Geometry: final body of the model. Coordinates: model frame, mm. Face numbers are marked on the shaded views. A direction names the side the tool comes from. Give positions to 0.01 mm unless a question says otherwise; leave off trailing zeros. Loops run counter-clockwise (first coordinate to the right, second up) from the corner with the lowest first, then second, coordinate; pieces in that order, holes last. Notation, with made-up numbers: (-20, 29.25) -> (18, 29.25) arc R21 ccw to (18, 60.25) -> close; hole circle Ø4 at (-4.5, -25.75). An arc over 180 degrees is marked (long way). One line per question, with ' | ' between items. Start each with the question number.
Item 1: Material intervals for line 1 along X through (y, z) = (8.75, -11.5); line 2 along X through (y, z) = (5.5, 0); line 3 along X through (y, z) = (8, -10), sorted ascending. Write a range as [from, to].
Item 2: Section B-B on x = 20.75. Return loops of the section in (y, z).
Item 3: Section D-D on z = 9.75. Return loops of the section in (x, y), then the cut area to 3 significant figures.
Item 4: Mould query, pull axis Z, two halves, no side actions, for the marked faces 1, 2, 3 and 4. Classes: released by +Z, released by -Z, zero draft, split by the parting line, or undercut.
Item 5: Section A-A on y = 6.5. Return loops of the section in (x, z).
Item 6: Section C-C on z = -1.75. Return loops of the section in (x, y), then the cut area to 3 significant figures.
Item 7: Set-up query: the marked faces 5, 6 and 7. Return all of +Z, -Z, +X, -X, +Y, -Y with unobstructed straight access to the full face (end or side cutting, diameter ignored); none if empty.
Item 8: Pin query (flat end, axial travel): P1, Ø3, axis at y = 11, z = -10.5, coming from the -X side; P2, Ø2.5, axis at y = 9.5, z = -6.5, coming from the -X side; P3, Ø3, axis at y = 11, z = 3.5, coming from the -X side; P4, Ø6.5, axis at x = 18.5, y = 8.5, coming from the +Z side. Return the tip coordinate at first contact, or that it passes through.
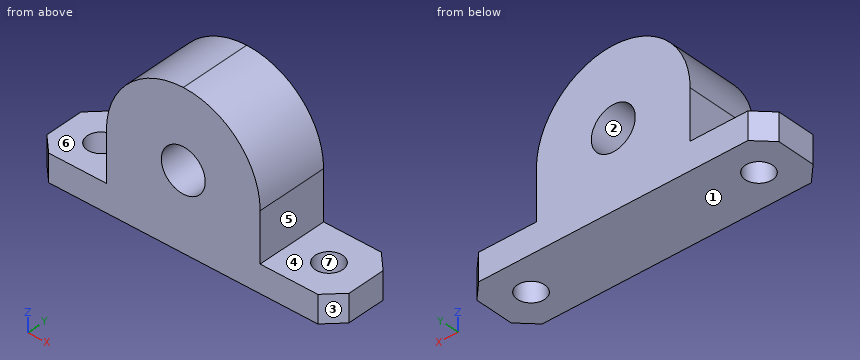
from build123d import *

# Parameters (mm, degrees)
SKETCH_1_R          = 4
EXTRUDE_1_DEPTH     = 13
CUT_EXTRUDE_1_REACH = 43.343
SKETCH_2_R          = 2.5
CHAMFER_1_SIZE      = 3


with BuildPart() as part:
    # 草图1 → 凸台-拉伸1 (new body)
    with BuildSketch(Plane(origin=(0, 0, 0), x_dir=(1, 0, 0), z_dir=(0, 1, 0))):
        with BuildLine():
            Line((-14, 0), (-14, 9))
            Line((-14, 9), (-27.5, 9))
            Line((-27.5, 9), (-27.5, 14))
            Line((-27.5, 14), (-14, 14))
            Line((-14, 14), (14, 14))
            Line((14, 14), (27.5, 14))
            Line((27.5, 14), (27.5, 9))
            Line((27.5, 9), (14, 9))
            Line((14, 9), (14, 0))
            ThreePointArc((14, 0), (9.899494937, -9.899494937), (0, -14))
            ThreePointArc((0, -14), (-9.899494937, -9.899494937), (-14, 0))
        make_face()
        with Locations(Location((0, 0, 0), (0, 0, 90))):
            Circle(SKETCH_1_R, mode=Mode.SUBTRACT)
    extrude(amount=EXTRUDE_1_DEPTH)

    # 草图2 → 切除-拉伸1 (cut, up to next)
    with BuildSketch(Plane(origin=(0, 0, -14), x_dir=(-1, 0, 0), z_dir=(0, 0, -1)), mode=Mode.PRIVATE) as cut_extrude_1_sk1:
        with Locations((-20.75, 6.5)):
            Circle(SKETCH_2_R)
    cut_extrude_1_tool1 = extrude(cut_extrude_1_sk1.sketch, amount=-CUT_EXTRUDE_1_REACH, mode=Mode.PRIVATE) & part.part
    # 草图2 → 切除-拉伸1 (cut, up to next)
    with BuildSketch(Plane(origin=(0, 0, -14), x_dir=(-1, 0, 0), z_dir=(0, 0, -1)), mode=Mode.PRIVATE) as cut_extrude_1_sk2:
        with Locations((20.75, 6.5)):
            Circle(SKETCH_2_R)
    cut_extrude_1_tool2 = extrude(cut_extrude_1_sk2.sketch, amount=-CUT_EXTRUDE_1_REACH, mode=Mode.PRIVATE) & part.part
    add(cut_extrude_1_tool1.solids().sort_by_distance((20.75, 6.5, -14))[0], mode=Mode.SUBTRACT)
    add(cut_extrude_1_tool2.solids().sort_by_distance((-20.75, 6.5, -14))[0], mode=Mode.SUBTRACT)

    # 倒角1
    chamfer_1_edges = [part.edges().sort_by_distance(p)[0] for p in [
        (-27.5, 0, -11.5),
        (27.5, 0, -11.5),
        (27.5, 13, -11.5),
        (-27.5, 13, -11.5),
    ]]
    chamfer(chamfer_1_edges, length=CHAMFER_1_SIZE)


solid = part.part
Result sheet:
1) line 1: x = [-27.5, -21.84], [-19.66, 19.66], [21.84, 27.5] | line 2: x = [-14, -4], [4, 14] | line 3: x = [-27.5, -22.75], [-18.75, 18.75], [22.75, 27.5]
2) outline: (0, -14) -> (4, -14) -> (4, -9) -> (0, -9) -> close; (9, -14) -> (13, -14) -> (13, -9) -> (9, -9) -> close
3) outline: (-10.05, 0) -> (10.05, 0) -> (10.05, 13) -> (-10.05, 13) -> close | area: 261 mm²
4) face 1: released by -Z | face 2: undercut | face 3: zero draft | face 4: released by +Z
5) outline: (-27.5, -14) -> (-23.25, -14) -> (-23.25, -9) -> (-27.5, -9) -> close; (-18.25, -14) -> (18.25, -14) -> (18.25, -9) -> (14, -9) -> (14, 0) arc R14 ccw to (-14, 0) -> (-14, -9) -> (-18.25, -9) -> close; (23.25, -14) -> (27.5, -14) -> (27.5, -9) -> (23.25, -9) -> close; hole circle Ø8 at (0, 0)
6) outline: (-14, 0) -> (-3.6, 0) -> (-3.6, 13) -> (-14, 13) -> close; (3.6, 0) -> (14, 0) -> (14, 13) -> (3.6, 13) -> close | area: 270 mm²
7) face 5: +Z, +X, +Y, -Y | face 6: +Z, -X, +Y, -Y | face 7: +Z, -Z
8) P1: stops at x = -27.5 | P2: stops at x = -14 | P3: stops at x = -13.86 | P4: stops at z = -9
